Geometry: final body of the model. Coordinates: model frame, mm. A direction names the side the tool comes from. Round coordinates to 2 decimals unless told otherwise and drop trailing zeros. Loops run counter-clockwise (first coordinate to the right, second up) from the corner with the lowest first, then second, coordinate; pieces in that order, holes last. Notation, with made-up numbers: (-12, -5.75) - (45, -5.75) arc R26 cw to (45, 11.25) - close; hole circle Ø1 at (74.25, -33). An arc over 180 degrees is marked (long way). Return JSON: item names as keys, results as strings. Group by question number.
1. Section D-D on z = 2. Return loops of the section in (x, y).
2. Material intervals for probe 1 along X at (y, z) = (-1.55, -1); probe 2 along Z at (x, y) = (3.25, -0.65); probe 3 along Y at (x, z) = (8.25, 1.3), sorted ascending.
3. Section B-B on z = 0. Return loops of the section in (x, y), and give its area (3 significant figures).
4. Section C-C on x = -1.25. Return loops of the section in (y, z).
5. Set-up query: faces 1 (the face through (5, 0, 3)), 2 (the face through (-0.8, -1, 0)). Return all of +Z, -Z, +X, -X, +Y, -Y with unobstructed straight access to the full face (end or side cutting, diameter ignored); none if empty.
6. Section A-A on y = 0. Return loops of the section in (x, z), and give its area (3 significant figures).
from build123d import *

# Parameters (mm, degrees)
SKETCH1_R           = 3
BOSS_EXTRUDE1_DEPTH = 10
SKETCH2_R           = 1.2
BOSS_EXTRUDE2_DEPTH = 0.8
SKETCH3_R           = 0.4
BOSS_EXTRUDE3_DEPTH = 3.2
SKETCH4_R           = 0.3
BOSS_EXTRUDE4_DEPTH = 1


with BuildPart() as part:
    # Sketch1 → Boss-Extrude1 (new body)
    with BuildSketch(Plane(origin=(0, 0, 0), x_dir=(0, 0, -1), z_dir=(1, 0, 0))):
        Circle(SKETCH1_R)
    extrude(amount=BOSS_EXTRUDE1_DEPTH)

    # Sketch2 → Boss-Extrude2 (add)
    with BuildSketch(Plane.ZY):
        Circle(SKETCH2_R)
    extrude(amount=BOSS_EXTRUDE2_DEPTH)

    # Sketch3 → Boss-Extrude3 (add)
    with BuildSketch(Plane.ZY.offset(0.8)):
        Circle(SKETCH3_R)
    extrude(amount=BOSS_EXTRUDE3_DEPTH)

    # Sketch4 → Boss-Extrude4 (add)
    with BuildSketch(Plane(origin=(10, 0, 0), x_dir=(0, 0, -1), z_dir=(1, 0, 0))):
        with Locations((-2, 0)):
            Circle(SKETCH4_R)
        with Locations((2, 0)):
            Circle(SKETCH4_R)
    extrude(amount=BOSS_EXTRUDE4_DEPTH)


solid = part.part
Taken from the geometry:
{
 "1": {"outline": "(0, -2.24) - (10, -2.24) - (10, -0.3) - (11, -0.3) - (11, 0.3) - (10, 0.3) - (10, 2.24) - (0, 2.24) - close"},
 "2": {"probe 1": "0 to 10", "probe 2": "-2.93 to 2.93", "probe 3": "-2.7 to 2.7"},
 "3": {"outline": "(-4, -0.4) - (-0.8, -0.4) - (-0.8, -1.2) - (0, -1.2) - (0, -3) - (10, -3) - (10, 3) - (0, 3) - (0, 1.2) - (-0.8, 1.2) - (-0.8, 0.4) - (-4, 0.4) - close", "area": "64.5 mm2"},
 "4": {"outline": "circle Ø0.8 at (0, 0)"},
 "5": {"face 1": "+X, -X", "face 2": "-X"},
 "6": {"outline": "(-4, -0.4) - (-0.8, -0.4) - (-0.8, -1.2) - (0, -1.2) - (0, -3) - (10, -3) - (10, -2.3) - (11, -2.3) - (11, -1.7) - (10, -1.7) - (10, 1.7) - (11, 1.7) - (11, 2.3) - (10, 2.3) - (10, 3) - (0, 3) - (0, 1.2) - (-0.8, 1.2) - (-0.8, 0.4) - (-4, 0.4) - close", "area": "65.7 mm2"}
}
